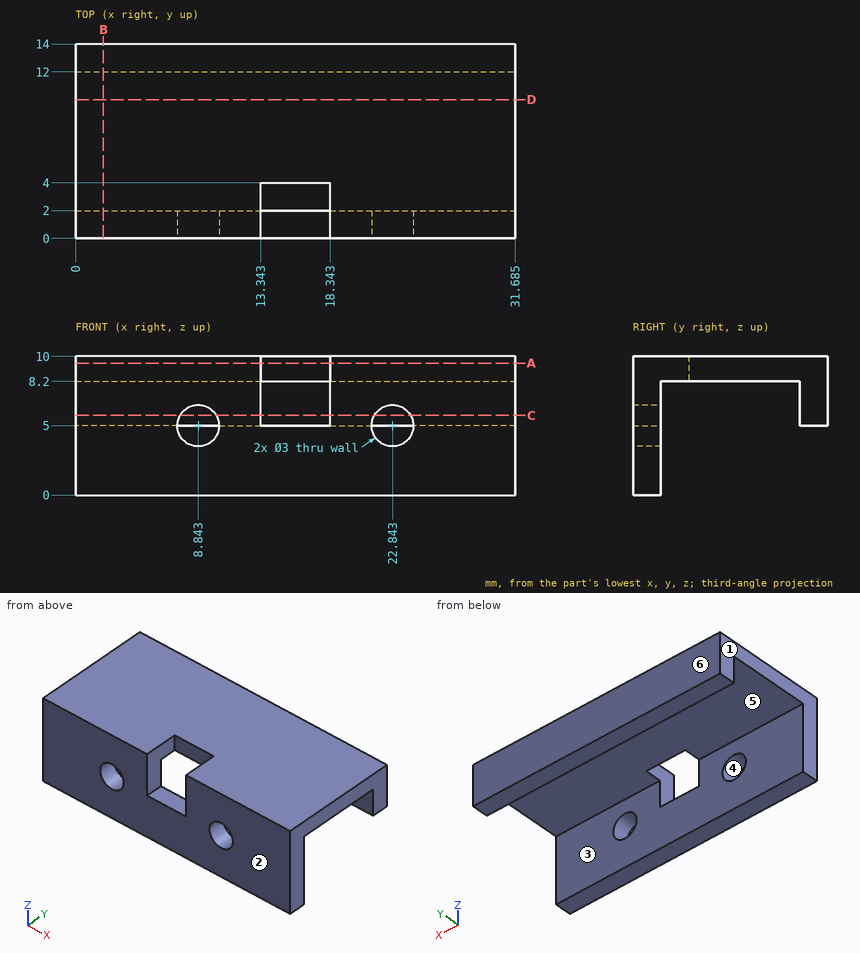
Study the drawing (mm; zero at the part's minimum x, y, z) and answer. A direction names the side the tool comes from. Give positions to 0.01 mm unless a question says otherwise; leave off trailing zeros. Order: outer loops, then holes, each group sorted by start corner. A loop starts at its lowest first (then second) coordinate and runs counter-clockwise, first axis right, second up. Notation, with made-up numbers: (5.25, 25) -> (36.25, 25) arc R11 ccw to (36.25, 45) -> close; hole circle Ø7 at (82.25, 35.5). An arc over 180 degrees is marked (long way). Write item = value, one per line.
1. A cutting plane is placed at C-C, the plane z = 5.75. Write down the section's boundary in (x, y) (1 decimal).
Numbers:
outline = (0, 0) -> (7.5, 0) -> (7.5, 2) -> (0, 2) -> close; (0, 12) -> (31.7, 12) -> (31.7, 14) -> (0, 14) -> close; (10.1, 0) -> (13.3, 0) -> (13.3, 2) -> (10.1, 2) -> close; (18.3, 0) -> (21.5, 0) -> (21.5, 2) -> (18.3, 2) -> close; (24.1, 0) -> (31.7, 0) -> (31.7, 2) -> (24.1, 2) -> close
2. A cutting plane is placed at B-B, the plane x = 2. Write down the section's boundary in (y, z), and give its area (3 significant figures).
Numbers:
outline = (0, 0) -> (2, 0) -> (2, 8.2) -> (12, 8.2) -> (12, 5) -> (14, 5) -> (14, 10) -> (0, 10) -> close
area = 48.0 mm²
3. The mould has two halves that part along Y. Classify the marked faces 1, 2 and 3: +Y half, -Y half, draft (parallel to the pull), parting line (faces both ways), or undercut.
Numbers:
face_1 = draft
face_2 = -Y half
face_3 = undercut
4. Given pin 1 (4 mm diameter, centred on y = 10.5, z = 3.5, fed in from -X); pin 2 (2 mm diameter, centred on x = 8.5, y = 12.5, fed in from -Z); pin 3 (2 mm diameter, centred on x = 16.5, z = 9.5, fed in from -Y); pin 4 (1.6 mm diameter, centred on x = 15.5, y = 1, fed in from +Z), each flat-ended and moving along its own axis, determine where each tip first touches the part or whether it passes through.
Numbers:
pin_1 = through
pin_2 = 5
pin_3 = 4
pin_4 = 5
5. For the marked faces 4, 5 and 6, determine the directions among +Z, -Z, +X, -X, +Y, -Y from which every point of the face is accessible in a straight line to the end or side of a thin tool.
Numbers:
face_4 = -Y
face_5 = -Z, +X, -X
face_6 = +Z, -Z, +X, -X, +Y
6. Straight lines are drawn through the part: line 1 along Y through (x, z) = (23.5, 8); line 2 along Z through (x, y) = (2, 11); line 3 along Y through (x, z) = (16.5, 6.25). For each, find the intervals that lie inside material, in ascending order.
Numbers:
line_1 = 0 to 2, 12 to 14
line_2 = 8.2 to 10
line_3 = 12 to 14
7. A cutting plane is placed at D-D, the plane y = 10. Write down the section's boundary in (x, z) (1 decimal).
Numbers:
outline = (0, 8.2) -> (31.7, 8.2) -> (31.7, 10) -> (0, 10) -> close
8. A cutting plane is placed at A-A, the plane z = 9.5. Write down the section's boundary in (x, y) (1 decimal).
Numbers:
outline = (0, 0) -> (13.3, 0) -> (13.3, 4) -> (18.3, 4) -> (18.3, 0) -> (31.7, 0) -> (31.7, 14) -> (0, 14) -> close
